Input: dimensioned drawing with shaded views. Units: mm. Origin: part minimum x, y, z. A direction names the side the tool comes from. Coordinates: 2 decimals unless noted, no trailing zeros. Order: outer loops, then holes, each group sorted by start corner. A loop starts at its lowest first (then second) coordinate and runs counter-clockwise, first axis right, second up. Notation, with made-up numbers: (57.25, 43) - (79.25, 43) arc R30 cw to (79.25, 75) - close; hole circle Ø5 at (72.5, 24). An arc over 180 degrees is marked (long way). Answer as CSV lines item,"result". Start each with the question number.
Item 1: Section B-B (y = 5). Output: boundary loops of the cut face in (x, z), and give its area (3 significant figures).
Item 2: Section A-A (z = 8.5). Output: boundary loops of the cut face in (x, y).
Item 3: Draft query along Z for the marked faces 1, 2, 3 and 4. Return one class per face: +Z half, -Z half, draft (parallel to the pull), parting line (faces both ways), or undercut.
Item 4: Section C-C (x = 36). Output: boundary loops of the cut face in (y, z).
Item 5: Access query for the marked faces 5 and 6. Directions: +Z, -Z, +X, -X, +Y, -Y. A direction counts if a zero-diameter tool reaches every point of the face in a straight line with its end or side. Return the directions, or none.
Item 6: Material intervals for line 1 along Y through (x, z) = (29, 1.5); line 2 along Z through (x, y) = (13.5, 7.25); line 3 along Y through (x, z) = (26.5, 6.25), sorted ascending.
Item 7: Section D-D (y = 8.5). Output: boundary loops of the cut face in (x, z), and give its area (3 significant figures).
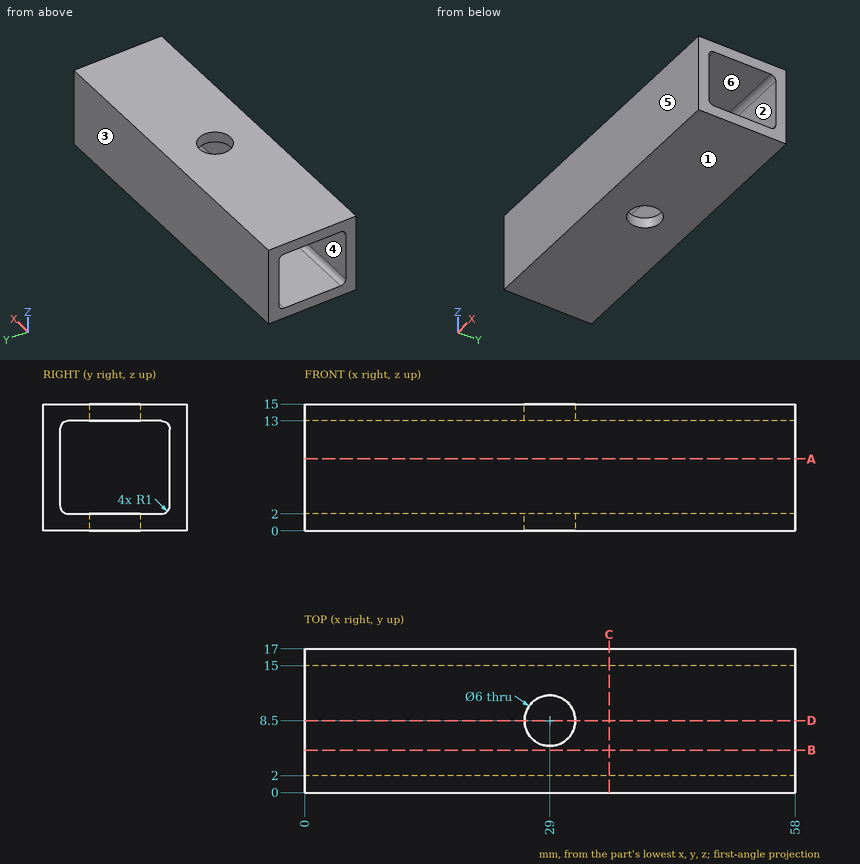
Determined:
1,outline,"(0, 0) - (58, 0) - (58, 2) - (0, 2) - close; (0, 13) - (58, 13) - (58, 15) - (0, 15) - close"
1,area,"232 mm^2"
2,outline,"(0, 0) - (58, 0) - (58, 2) - (0, 2) - close; (0, 15) - (58, 15) - (58, 17) - (0, 17) - close"
3,face 1,"-Z half"
3,face 2,"undercut"
3,face 3,"draft"
3,face 4,"undercut"
4,outline,"(0, 0) - (17, 0) - (17, 15) - (0, 15) - close; hole (2, 3) arc R1 ccw to (3, 2) - (14, 2) arc R1 ccw to (15, 3) - (15, 12) arc R1 ccw to (14, 13) - (3, 13) arc R1 ccw to (2, 12) - close"
5,face 5,"+Z, -Z, +X, -X, -Y"
5,face 6,"+X, -X"
6,line 1,"y = 0 to 5.5, 11.5 to 17"
6,line 2,"z = 0 to 2, 13 to 15"
6,line 3,"y = 0 to 2, 15 to 17"
7,outline,"(0, 0) - (26, 0) - (26, 2) - (0, 2) - close; (0, 13) - (26, 13) - (26, 15) - (0, 15) - close; (32, 0) - (58, 0) - (58, 2) - (32, 2) - close; (32, 13) - (58, 13) - (58, 15) - (32, 15) - close"
7,area,"208 mm^2"
